from build123d import *

# Parameters (mm, degrees)
F0_W            = 225
F0_H            = 210
F1_DEPTH        = 25
F3_DEPTH        = 95
F4_R            = 37.5
F5_DEPTH        = 10
F5_DEPTH_BACK   = 127
F6_R            = 40
F7_DEPTH        = 10
F7_DEPTH_BACK   = 127
F8_W            = 60
F8_H            = 60
F9_DEPTH        = 10
F10_R           = 10
F12_DEPTH       = 15
F14_D           = 15
F14_CBORE_D     = 30
F14_CBORE_DEPTH = 10
F15_R           = 10
F16_R           = 19.5
F17_DEPTH       = 220.001
F18_R           = 19.5
F19_DEPTH       = 235.001


with BuildPart() as f1:
    # F0 (on Top) → F1 (new body)
    with BuildSketch(Plane.XY):
        Rectangle(F0_W, F0_H)
    extrude(amount=F1_DEPTH)

    # F2 (on face) → F3 (join)
    with BuildSketch(Plane.XY.offset(25)):
        with BuildLine():
            Line((-63.5, -25), (-63.5, -105))
            Line((-63.5, -105), (-48.5, -105))
            Line((-48.5, -105), (-48.5, -38.981817))
            ThreePointArc((-48.5, -38.981817), (14.988853, -7.488853), (46.481817, 56))
            Line((46.481817, 56), (112.5, 56))
            Line((112.5, 56), (112.5, 71))
            Line((112.5, 71), (32.5, 71))
            ThreePointArc((32.5, 71), (4.382251, 3.117749), (-63.5, -25))
        make_face()
    extrude(amount=F3_DEPTH)

    # F4 (on face) → F5 (join, two sides)
    with BuildSketch(Plane.XZ.offset(105)) as f5_sk:
        with Locations((-56, 120)):
            Circle(F4_R)
    extrude(amount=F5_DEPTH)
    extrude(f5_sk.sketch, amount=-F5_DEPTH_BACK)

    # F6 (on face) → F7 (join, two sides)
    with BuildSketch(Plane.YZ.offset(112.5)) as f7_sk:
        with Locations((63.5, 120)):
            Circle(F6_R)
    extrude(amount=F7_DEPTH)
    extrude(f7_sk.sketch, amount=-F7_DEPTH_BACK)

    # F8 (on face) → F9 (join)
    with BuildSketch(Plane.XY.offset(25)):
        with Locations((82.5, -75)):
            Rectangle(F8_W, F8_H)
    extrude(amount=F9_DEPTH)

    # F10
    f10_edges = [f1.edges().sort_by_distance(p)[0] for p in [
        (52.5, -45, 30),
    ]]
    fillet(f10_edges, radius=F10_R)

    # F11 (on face) → F12 (cut)
    with BuildSketch(Plane.XY.offset(25)):
        with BuildLine():
            ThreePointArc((54.075507, 47.000001), (21.352813, -13.852813), (-39.500001, -46.575507))
            Line((-39.500001, -46.575507), (-39.500001, -96.000001))
            Line((-39.500001, -96.000001), (43.500001, -96.000001))
            Line((43.500001, -96.000001), (43.500001, -55))
            ThreePointArc((43.500001, -55), (49.064972, -41.564972), (62.5, -36.000001))
            Line((62.5, -36.000001), (103.500001, -36.000001))
            Line((103.500001, -36.000001), (103.500001, 47.000001))
            Line((103.500001, 47.000001), (54.075507, 47.000001))
        make_face()
    extrude(amount=-F12_DEPTH, mode=Mode.SUBTRACT)

    # F14 (through all)
    with Locations(Plane.XY.offset(35)):
        with Locations((82.5, -75)):
            CounterBoreHole(F14_D / 2, F14_CBORE_D / 2, F14_CBORE_DEPTH)

    # F15
    f15_edges = [f1.edges().sort_by_distance(p)[0] for p in [
        (103.500001, -36.000001, 17.5),
        (43.500001, -96.000001, 17.5),
        (-39.500001, -46.575507, 17.5),
        (54.075507, 47.000001, 17.5),
        (-39.500001, -96.000001, 17.5),
        (103.500001, 47.000001, 17.5),
    ]]
    fillet(f15_edges, radius=F15_R)

    # F16 (on face) → F17 (cut, through all)
    with BuildSketch(Plane.XZ.offset(115)):
        with Locations((-56, 120)):
            Circle(F16_R)
    extrude(amount=-F17_DEPTH, mode=Mode.SUBTRACT)

    # F18 (on face) → F19 (cut, through all)
    with BuildSketch(Plane.YZ.offset(122.5)):
        with Locations((63.5, 120)):
            Circle(F18_R)
    extrude(amount=-F19_DEPTH, mode=Mode.SUBTRACT)


solid = f1.part
CAD build for the part. Positions are in the model's coordinates, mm. A direction names the side the tool comes from. Give positions to 0.01 mm unless a question says otherwise; leave off trailing zeros. Order: outer loops, then holes, each group sorted by start corner. A loop starts at its lowest first (then second) coordinate and runs counter-clockwise, first axis right, second up. Notation, with made-up numbers: (45, 46.5) -> (56, 46.5) arc R24 cw to (56, 84.5) -> close; hole circle Ø9 at (-33, 88.5). An arc over 180 degrees is marked (long way). Return JSON: item names as keys, results as strings.
Q1. Mould opens along Y. For faces 6 (the face through (100.49, -33.15, 17.4)), 7 (the face through (-37.39, -48.33, 17.4)), 8 (the face through (52.5, -80, 30)), 9 (the face through (-40, -115, 104)) say: pulls with the +Y half, pulls with the -Y half, needs draft (parallel to the pull), parting line crosses it, or undercut.
Working result:
{"face 6": "undercut", "face 7": "undercut", "face 8": "needs draft", "face 9": "pulls with the -Y half"}
Q2. Saw through at A-A (z = 28.5). Write the cut outline in (x, y), then the cut area to 3 significant figures.
Working result:
{"outline": "(-63.5, -105) -> (-48.5, -105) -> (-48.5, -38.98) arc R111 ccw to (46.48, 56) -> (112.5, 56) -> (112.5, 71) -> (32.5, 71) arc R96 cw to (-63.5, -25) -> close; (52.5, -105) -> (112.5, -105) -> (112.5, -45) -> (62.5, -45) arc R10 ccw to (52.5, -55) -> close; hole circle Ø30 at (82.5, -75)", "area": "7,270 mm²"}
Q3. Flat gauge pins, fed straight in: pin 1 (2 mm diameter, centred on x = -24.5, z = 105.5, fed in from +Y); pin 2 (17.5 mm diameter, centred on y = -64, z = 57, fed in from +X); pin 3 (8 mm diameter, centred on x = 55, y = 10, fed in from +Z). Where does each tip first touch, or does it go through?
Working result:
{"pin 1": "y = 22", "pin 2": "x = -48.5", "pin 3": "z = 10"}
Q4. Drill centre lines: line 1 (Y direction, x = 82, z = 28); line 2 (Y direction, x = 82, z = 19); line 3 (Z direction, x = 88, y = 63). Where is each one in solid material? Low to high.
Working result:
{"line 1": "-105 to -89.99, -60.01 to -45, 56 to 71", "line 2": "-105 to -82.48, -67.52 to -36, 47 to 105", "line 3": "0 to 100.51, 139.49 to 160"}
Q5. Saw through at D-D (y = -99.5). Write the cut outline in (x, z).
Working result:
{"outline": "(-112.5, 0) -> (112.5, 0) -> (112.5, 35) -> (52.5, 35) -> (52.5, 25) -> (-48.5, 25) -> (-48.5, 83.26) arc R37.5 ccw (long way) to (-63.5, 83.26) -> (-63.5, 25) -> (-112.5, 25) -> close; hole circle Ø39 at (-56, 120)"}
Q6. Saw through at C-C (y = -3). Write the cut outline in (x, z), then the cut area to 3 significant figures.
Working result:
{"outline": "(-112.5, 0) -> (112.5, 0) -> (112.5, 25) -> (103.5, 25) -> (103.5, 10) -> (30.97, 10) -> (30.97, 25) -> (19.23, 25) -> (19.23, 120) -> (-2.34, 120) -> (-2.34, 25) -> (-112.5, 25) -> close; circle Ø75 at (-56, 120); hole circle Ø39 at (-56, 120)", "area": "9,810 mm²"}
Q7. Which spindle directions (+Z, -Z, +X, -X, +Y, -Y) get a long thin tool onto all of the face, cutting with end or side? Do faces 1 (the face through (-2, -105, 23)), 2 (the face through (87, -45, 30)), 3 (the face through (55.83, 44.89, 17.4)), 4 (the face through (86, -68, 25)), 5 (the face through (14.27, -8.2, 71.84)). Say none if no direction does.
Working result:
{"face 1": "-Z, +X, -X, -Y", "face 2": "+Z, +X", "face 3": "none", "face 4": "+Z", "face 5": "+X, -Y"}
Q8. Saw through at B-B (x = 82.5). Write the cut outline in (y, z).
Working result:
{"outline": "(-105, 0) -> (-82.5, 0) -> (-82.5, 25) -> (-90, 25) -> (-90, 35) -> (-105, 35) -> close; (-67.5, 0) -> (105, 0) -> (105, 25) -> (71, 25) -> (71, 80.71) arc R40 ccw (long way) to (56, 80.71) -> (56, 25) -> (47, 25) -> (47, 10) -> (-36, 10) -> (-36, 25) -> (-45, 25) -> (-45, 35) -> (-60, 35) -> (-60, 25) -> (-67.5, 25) -> close; hole circle Ø39 at (63.5, 120)"}
